from build123d import *

# Parameters (mm, degrees)
BOSS_EXTRUDE1_DEPTH  = 200.66
SKETCH2_W            = 9.525
SKETCH2_H            = 12.7
CUT_EXTRUDE1_DEPTH   = 4.175
M3_CLEARANCE_HOLE1_D = 3.4


with BuildPart() as part:
    # Sketch1 → Boss-Extrude1 (new body)
    with BuildSketch(Plane.XY):
        Polygon((0, 0), (0, 12.7), (3.175, 12.7), (3.175, 3.175), (12.7, 3.175), (12.7, 0), align=None)
    extrude(amount=BOSS_EXTRUDE1_DEPTH)

    # Sketch2 → Cut-Extrude1 (cut, through all)
    with BuildSketch(Plane(origin=(0, 3.175, 0), x_dir=(1, 0, 0), z_dir=(0, 1, 0))):
        with Locations((7.9375, -6.35)):
            Rectangle(SKETCH2_W, SKETCH2_H)
        with Locations((7.9375, -194.31)):
            Rectangle(SKETCH2_W, SKETCH2_H)
    extrude(amount=-CUT_EXTRUDE1_DEPTH, mode=Mode.SUBTRACT)

    # M3 Clearance Hole1 (through all)
    with Locations(Plane(origin=(0, 6.35, 6.35), x_dir=(0, 0, -1), z_dir=(-1, 0, 0))):
        with Locations((0, 0), (-187.96, 0)):
            Hole(M3_CLEARANCE_HOLE1_D / 2)


solid = part.part
Verification items for the finished model (mm, model axes). A direction names the side the tool comes from. Coordinates: 2 decimals unless noted, no trailing zeros. Order: outer loops, then holes, each group sorted by start corner. A loop starts at its lowest first (then second) coordinate and runs counter-clockwise, first axis right, second up. Notation, with made-up numbers: (-5, -20.5) -> (37, -20.5) arc R7 ccw to (37, -7.5) -> close; hole circle Ø10 at (-39, 62). An arc over 180 degrees is marked (long way). Put each result on its own line as item: value. Start each with the question number.
1. Cross-section at A-A, the plane y = 6.35. Record the boundary of the cut face in (x, z) (3 decimals), then the cut area to 3 significant figures.
2. Material ranges on L1, parallel to Z at x = 2.55, y = 6.35; L2, parallel to Y at x = 2.15, z = 6.35; L3, parallel to X at y = 12, z = 21.5 (3 decimals), recorded low to high. Write a range as [from, to].
3. Cross-section at B-B, the plane z = 194.31. Record the boundary of the cut face in (x, y) (3 decimals), then the cut area to 3 significant figures.
4. Access from +Z, -Z, +X, -X, +Y, -Y to the whole of each face (thin tool, end or side, straight path). Record for faces 4 (the flat face through (8, 2, 12.7)), 5 (the flat face through (8, 3.175, 99)), 6 (the flat face through (2, 6, 0)).
5. Go/stop test with flat-tipped pins: pin 1 Ø1.6 at (x, y) = (9, 1.5) entering from +Z; pin 2 Ø2.5 at (x, y) = (8.5, 2) entering from -Z; pin 3 Ø5.5 at (y, z) = (6.35, 6.35) entering from +X (3 decimals). Record where each tip stops, or that it passes through.
6. Cross-section at D-D, the plane z = 141.5. Record the boundary of the cut face in (x, y) (3 decimals).
7. Cross-section at C-C, the plane x = 7. Record the boundary of the cut face in (y, z) (3 decimals).
8. Mould release check, pull along Z, two halves, no side actions. Record for faces 1 (the flat face through (6, 0, 99)), 2 (the cylindrical face through (1.6, 5.2, 5.1)), 3 (the flat face through (8, 2, 187.96)): released by +Z, released by -Z, zero draft, split by the parting line, or undercut.
Computed:
1. outline: (0, 0) -> (3.175, 0) -> (3.175, 4.65) -> (0, 4.65) -> close; (0, 8.05) -> (3.175, 8.05) -> (3.175, 192.61) -> (0, 192.61) -> close; (0, 196.01) -> (3.175, 196.01) -> (3.175, 200.66) -> (0, 200.66) -> close
1. area: 616 mm2
2. L1: [0, 4.65], [8.05, 192.61], [196.01, 200.66]
2. L2: [0, 4.65], [8.05, 12.7]
2. L3: [0, 3.175]
3. outline: (0, 0) -> (3.175, 0) -> (3.175, 4.65) -> (0, 4.65) -> close; (0, 8.05) -> (3.175, 8.05) -> (3.175, 12.7) -> (0, 12.7) -> close
3. area: 29.5 mm2
4. face 4: -Z, +X, +Y, -Y
4. face 5: +Z, -Z, +X, +Y
4. face 6: -Z, +X, -X, +Y, -Y
5. pin 1: z = 187.96
5. pin 2: z = 12.7
5. pin 3: x = 3.175
6. outline: (0, 0) -> (12.7, 0) -> (12.7, 3.175) -> (3.175, 3.175) -> (3.175, 12.7) -> (0, 12.7) -> close
7. outline: (0, 12.7) -> (3.175, 12.7) -> (3.175, 187.96) -> (0, 187.96) -> close
8. face 1: zero draft
8. face 2: undercut
8. face 3: released by +Z
